The model under review builds one solid part; all positions refer to its coordinate system, in mm. A direction names the side the tool comes from. Round coordinates to 2 decimals unless told otherwise and drop trailing zeros. Write each loop counter-clockwise with the first axis right and the second up, starting at its lowest first coordinate (ties: lowest second). Pieces come first, ordered by that corner, then holes. Notation, with made-up numbers: (79, 54.5) -> (99, 54.5) arc R16 cw to (99, 83.5) -> close; hole circle Ø9 at (-26.5, -25.5). An arc over 180 degrees is marked (long way). Return JSON: item names as keys, results as strings. Group by question number.
1. Take a section at B-B, the plane y = 3. Write out the cut boundary in (x, z) (3 decimals).
2. Take a section at C-C, the plane z = 0.5. Write out the cut boundary in (x, y) (3 decimals), then the cut area to 3 significant figures.
3. Take a section at D-D, the plane z = 8. Write out the cut boundary in (x, y) (3 decimals).
4. For line 1 along Y through (x, z) = (17.5, 4.9); line 2 along X through (y, z) = (-2.5, 2.5); line 3 along X through (y, z) = (0.5, 1.75) (3 decimals), list the stretches that pass through material, from the lowest coordinate up. Write a range as from..to.
5. Tool access review of faces 1 (the flat face through (-15.5, 1, 5)), 2 (the flat face through (-18, 1, 6.45)), 3 (the flat face through (-15, -0.8, 4)), 4 (the flat face through (-18, 0, 5.35)): name each direction out of +Z, -Z, +X, -X, +Y, -Y from which nothing blocks a thin tool from reaching the whole face with its end or side.
6. Clearance check with flat-ended pins moving along their axes: P1, Ø1.3, axis at x = 17.5, y = 2.65, coming from the -Z side; P2, Ø3.5, axis at x = 18, y = 3, coming from the +Z side; P3, Ø0.6, axis at x = 13, y = 3, coming from the -Z side; P4, Ø1, axis at x = -16, z = 5.5, coming from the +Y side. State where each tip first meets the part, or that it passes through.
7. Take a section at A-A, the plane x = 8. Write out the cut boundary in (y, z).
8. Mouldability with a two-part tool opening along Y and no side actions: class faces 5 (the cylindrical face through (0, -4, 8)), 6 (the flat face through (-17.6, -2, 4)), 7 (the flat face through (15.5, 1, 5)), 8 (the flat face through (19, 4.65, 5)) as pulls with the +Y half, pulls with the -Y half, needs draft (parallel to the pull), parting line crosses it, or undercut.
from build123d import *

# Parameters (mm, degrees)
BOSS_EXTRUDE1_DEPTH     = 20
SKETCH2_W               = 27.75
SKETCH2_H               = 8
BOSS_EXTRUDE2_DEPTH     = 4
CUT_EXTRUDE1_DEPTH      = 12.625
CUT_EXTRUDE1_DEPTH_BACK = 12.625
SKETCH6_W               = 4.5
SKETCH6_H               = 2.85
BOSS_EXTRUDE3_DEPTH     = 4.65
FILLET1_R               = 2
CUT_EXTRUDE2_REACH      = 23.586
SKETCH7_R               = 1.05
FILLET1_OF_MIRROR1_R    = 2
CUT_EXTRUDE3_START      = -16.5
CUT_EXTRUDE3_DEPTH      = 32
SHELL1_OUTLINE_W        = 2.3
SHELL1_OUTLINE_H        = 2.8
SHELL1_OUTLINE_W_2      = 1.3
SHELL1_DEPTH            = 5
SHELL1_START            = 4.7
SHELL1_2_DEPTH          = 0.65
SHELL1_START_2          = 16.6
SHELL1_3_DEPTH          = 2.3
SHELL1_START_3          = -18.9
SHELL1_4_DEPTH          = 1.3
SHELL1_START_4          = -17.6
SHELL1_5_DEPTH          = 34.2


with BuildPart() as part:
    # Sketch1 → Boss-Extrude1 (new, symmetric)
    with BuildSketch(Plane(origin=(0, 0, 0), x_dir=(0, 0, -1), z_dir=(1, 0, 0))):
        with BuildLine():
            Line((-10, 0), (0, 0))
            Line((0, 0), (0, -5))
            Line((0, -5), (-5, -5))
            ThreePointArc((-5, -5), (-8.535533906, -3.535533906), (-10, 0))
        make_face()
    extrude(amount=BOSS_EXTRUDE1_DEPTH, both=True)

    # Sketch2 → Boss-Extrude2 (add)
    with BuildSketch(Plane(origin=(0, 0, 0), x_dir=(1, 0, 0), z_dir=(0, 1, 0))):
        with Locations((0, -5)):
            Rectangle(SKETCH2_W, SKETCH2_H)
    extrude(amount=BOSS_EXTRUDE2_DEPTH)

    # Sketch4 → Cut-Extrude1 (cut, two sides: drawn at the far end of the back side and taken through both)
    with BuildSketch(Plane(origin=(0, 0, 0), x_dir=(0, 0, -1), z_dir=(1, 0, 0)).offset(-CUT_EXTRUDE1_DEPTH_BACK)):
        Polygon((-1, -0.8), (0, -0.8), (0, 4), (-7.4, 4), (-7.4, -0.8), align=None)
        with BuildLine():
            Line((-6.556434465, -3.161562797), (0, -4.2))
            Line((0, -4.2), (0, -0.8))
            Line((0, -0.8), (-1, -0.8))
            Line((-1, -0.8), (-7.4, -0.8))
            Line((-7.4, -0.8), (-7.4, -2.173874456))
            ThreePointArc((-7.4, -2.173874456), (-7.160405966, -2.823322504), (-6.556434465, -3.161562797))
        make_face()
    extrude(amount=CUT_EXTRUDE1_DEPTH + CUT_EXTRUDE1_DEPTH_BACK, mode=Mode.SUBTRACT)

    # Sketch6 → Boss-Extrude3 (add)
    with BuildSketch(Plane(origin=(0, 0, 0), x_dir=(1, 0, 0), z_dir=(0, 1, 0))):
        with Locations((-17.75, -5.025)):
            Rectangle(SKETCH6_W, SKETCH6_H)
    boss_extrude3 = extrude(amount=BOSS_EXTRUDE3_DEPTH)

    # Fillet1
    fillet1_edges = [part.edges().sort_by_distance(p)[0] for p in [
        (-15.5, 4.65, 5.025),
    ]]
    fillet(fillet1_edges, radius=FILLET1_R)

    # Sketch7 → Cut-Extrude2 (cut, up to next)
    with BuildSketch(Plane(origin=(0, 0, 3.6), x_dir=(-1, 0, 0), z_dir=(0, 0, -1)), mode=Mode.PRIVATE) as cut_extrude2_sk1:
        with Locations(Location((17.5, 2.65, 0), (0, 0, 90))):
            Circle(SKETCH7_R)
    cut_extrude2_tool1 = extrude(cut_extrude2_sk1.sketch, amount=-CUT_EXTRUDE2_REACH, mode=Mode.PRIVATE) & part.part
    cut_extrude2 = cut_extrude2_tool1.solids().sort_by_distance((-17.5, 2.65, 3.6))[0]
    add(cut_extrude2, mode=Mode.SUBTRACT)

    # Mirror1: Boss-Extrude3, Cut-Extrude2 across plane
    add(boss_extrude3.mirror(Plane(origin=(0, 0, 0), x_dir=(0, 0, 1), z_dir=(1, 0, 0))))
    add(cut_extrude2.mirror(Plane(origin=(0, 0, 0), x_dir=(0, 0, 1), z_dir=(1, 0, 0))), mode=Mode.SUBTRACT)

    # Fillet1 of Mirror1
    fillet1_of_mirror1_edges = [part.edges().sort_by_distance(p)[0] for p in [
        (15.5, 4.65, 5.025),
    ]]
    fillet(fillet1_of_mirror1_edges, radius=FILLET1_OF_MIRROR1_R)

    # Sketch4<3> → Cut-Extrude3 (cut)
    with BuildSketch(Plane(origin=(0, 0, 0), x_dir=(0, 0, -1), z_dir=(1, 0, 0)).offset(CUT_EXTRUDE3_START)):
        with BuildLine():
            Line((-6.556434465, -3.161562797), (0, -4.2))
            Line((0, -4.2), (0, -0.8))
            Line((0, -0.8), (-1, -0.8))
            Line((-1, -0.8), (-7.4, -0.8))
            Line((-7.4, -0.8), (-7.4, -2.173874456))
            ThreePointArc((-7.4, -2.173874456), (-7.160405966, -2.823322504), (-6.556434465, -3.161562797))
        make_face()
    extrude(amount=CUT_EXTRUDE3_DEPTH, mode=Mode.SUBTRACT)

    # Shell1: read off the stored shape, not the designer's step
    # Shell1 outline → Shell1 (cut)
    with BuildSketch(Plane.XY):
        with Locations((17.75, -2.5)):
            Rectangle(SHELL1_OUTLINE_W, SHELL1_OUTLINE_H)
        with Locations((-18.25, -2.5)):
            Rectangle(SHELL1_OUTLINE_W_2, SHELL1_OUTLINE_H)
    extrude(amount=SHELL1_DEPTH, mode=Mode.SUBTRACT)

    # Shell1 2 outline → Shell1 2 (cut)
    with BuildSketch(Plane.XY.offset(SHELL1_START)):
        with BuildLine():
            Line((16.6, 0.697437581), (16.6, -1.1))
            Line((16.6, -1.1), (18.9, -1.1))
            Line((18.9, -1.1), (18.9, 1.018283113))
            ThreePointArc((18.9, 1.018283113), (17.797044549, 0.520618743), (16.6, 0.697437581))
        make_face()
        with BuildLine():
            Line((-16.6, 0.3), (-16.6, 0.697437581))
            ThreePointArc((-16.6, 0.697437581), (-17.797044549, 0.520618743), (-18.9, 1.018283113))
            Line((-18.9, 1.018283113), (-18.9, -1.1))
            Line((-18.9, -1.1), (-17.6, -1.1))
            Line((-17.6, -1.1), (-17.6, 0.3))
            Line((-17.6, 0.3), (-16.6, 0.3))
        make_face()
    extrude(amount=SHELL1_2_DEPTH, mode=Mode.SUBTRACT)

    # Shell1 3 outline → Shell1 3 (cut)
    with BuildSketch(Plane.YZ.offset(SHELL1_START_2)):
        with BuildLine():
            Line((-3.9, 5), (-1.1, 5))
            Line((-1.1, 5), (-1.1, 8.741657387))
            ThreePointArc((-1.1, 8.741657387), (-3.122498999, 7.336664289), (-3.9, 5))
        make_face()
    extrude(amount=SHELL1_3_DEPTH, mode=Mode.SUBTRACT)

    # Shell1 4 outline → Shell1 4 (cut)
    with BuildSketch(Plane.YZ.offset(SHELL1_START_3)):
        with BuildLine():
            Line((-3.9, 5), (-1.1, 5))
            Line((-1.1, 5), (-1.1, 8.741657387))
            ThreePointArc((-1.1, 8.741657387), (-3.122498999, 7.336664289), (-3.9, 5))
        make_face()
    extrude(amount=SHELL1_4_DEPTH, mode=Mode.SUBTRACT)

    # Shell1 5 outline → Shell1 5 (cut)
    with BuildSketch(Plane.YZ.offset(SHELL1_START_4)):
        with BuildLine():
            ThreePointArc((-1.1, 8.741657387), (-1.415399361, 8.63409475), (-1.720465053, 8.5))
            Line((-1.720465053, 8.5), (-1.1, 8.5))
            Line((-1.1, 8.5), (-1.1, 8.741657387))
        make_face()
    extrude(amount=SHELL1_5_DEPTH, mode=Mode.SUBTRACT)


solid = part.part
Output:
{
 "1": {"outline": "(-20, 3.6) -> (-18.49, 3.6) -> (-18.49, 6.45) -> (-20, 6.45) -> close; (-16.51, 3.6) -> (-15.531, 3.6) -> (-15.531, 6.45) -> (-16.51, 6.45) -> close; (-13.875, 1) -> (-12.625, 1) -> (-12.625, 7.4) -> (12.625, 7.4) -> (12.625, 1) -> (13.875, 1) -> (13.875, 9) -> (-13.875, 9) -> close; (15.531, 3.6) -> (16.51, 3.6) -> (16.51, 6.45) -> (15.531, 6.45) -> close; (18.49, 3.6) -> (20, 3.6) -> (20, 6.45) -> (18.49, 6.45) -> close"},
 "2": {"outline": "(-20, -5) -> (20, -5) -> (20, 0) -> (12.625, 0) -> (12.625, -0.8) -> (15.5, -0.8) -> (15.5, -4.121) -> (-16.5, -4.121) -> (-16.5, -0.8) -> (-12.625, -0.8) -> (-12.625, 0) -> (-20, 0) -> close; hole (-18.9, -3.9) -> (-17.6, -3.9) -> (-17.6, -1.1) -> (-18.9, -1.1) -> close; hole (16.6, -3.9) -> (18.9, -3.9) -> (18.9, -1.1) -> (16.6, -1.1) -> close", "area": "63.5 mm^2"},
 "3": {"outline": "(-20, -4) -> (20, -4) -> (20, 0) -> (13.875, 0) -> (13.875, 4) -> (-13.875, 4) -> (-13.875, 0) -> (-20, 0) -> close; hole (-18.9, -2.492) -> (-17.6, -2.492) -> (-17.6, -1.1) -> (-18.9, -1.1) -> close; hole (16.6, -2.492) -> (18.9, -2.492) -> (18.9, -1.1) -> (16.6, -1.1) -> close"},
 "4": {"line 1": "y = -5..-3.9, 0.5..1.6, 3.7..4.65", "line 2": "x = -20..-18.9, -17.6..-16.5, 15.5..16.6, 18.9..20", "line 3": "x = -13.875..-12.625, 12.625..13.875"},
 "5": {"face 1": "+Z, -Z, +Y", "face 2": "+Z, -X, +Y", "face 3": "-Z", "face 4": "none"},
 "6": {"P1": "passes through", "P2": "stops at z = 6.45", "P3": "stops at z = 1", "P4": "stops at y = 4.38"},
 "7": {"outline": "(-5, 0) -> (-4.2, 0) -> (-3.16, 6.56) arc R1 cw to (-2.17, 7.4) -> (4, 7.4) -> (4, 9) -> (0, 9) -> (0, 10) arc R5 ccw to (-5, 5) -> close; hole (-1.72, 8.5) -> (-1.1, 8.5) -> (-1.1, 8.74) arc R3.9 ccw to start"},
 "8": {"face 5": "pulls with the -Y half", "face 6": "undercut", "face 7": "needs draft", "face 8": "pulls with the +Y half"}
}
